from build123d import *

# Parameters (mm, degrees)
F2_DEPTH = 1
F1_R     = 0.25
F3_DEPTH = 25


with BuildPart() as f2:
    # F0 (on Top) → F2 (new body)
    with BuildSketch(Plane.XY):
        with BuildLine():
            ThreePointArc((30.5, 6.5), (28.010408, 12.510408), (22, 15))
            Line((22, 15), (-22, 15))
            ThreePointArc((-22, 15), (-28.010408, 12.510408), (-30.5, 6.5))
            Line((-30.5, 6.5), (-30.5, -6.5))
            ThreePointArc((-30.5, -6.5), (-28.010408, -12.510408), (-22, -15))
            Line((-22, -15), (22, -15))
            ThreePointArc((22, -15), (28.010408, -12.510408), (30.5, -6.5))
            Line((30.5, -6.5), (30.5, 6.5))
        make_face()
    extrude(amount=F2_DEPTH)

    # F1 (on face) → F3 (cut)
    with BuildSketch(Plane.XY):
        with Locations((-27.111111, 12)):
            Circle(F1_R)
        with Locations((-27.111111, 6)):
            Circle(F1_R)
        with Locations((-27.111111, 0)):
            Circle(F1_R)
        with Locations((-27.111111, -6)):
            Circle(F1_R)
        with Locations((-27.111111, -12)):
            Circle(F1_R)
        with Locations((-20.333333, 12)):
            Circle(F1_R)
        with Locations((-20.333333, 6)):
            Circle(F1_R)
        with Locations((-20.333333, 0)):
            Circle(F1_R)
        with Locations((-20.333333, -6)):
            Circle(F1_R)
        with Locations((-20.333333, -12)):
            Circle(F1_R)
        with Locations((-13.555556, 12)):
            Circle(F1_R)
        with Locations((-13.555556, 6)):
            Circle(F1_R)
        with Locations((-13.555556, 0)):
            Circle(F1_R)
        with Locations((-13.555556, -6)):
            Circle(F1_R)
        with Locations((-13.555556, -12)):
            Circle(F1_R)
        with Locations((-6.777778, 12)):
            Circle(F1_R)
        with Locations((-6.777778, 6)):
            Circle(F1_R)
        with Locations((-6.777778, 0)):
            Circle(F1_R)
        with Locations((-6.777778, -6)):
            Circle(F1_R)
        with Locations((-6.777778, -12)):
            Circle(F1_R)
        with Locations((0, 12)):
            Circle(F1_R)
        with Locations((0, 6)):
            Circle(F1_R)
        with Locations((0, 0)):
            Circle(F1_R)
        with Locations((0, -6)):
            Circle(F1_R)
        with Locations((0, -12)):
            Circle(F1_R)
        with Locations((6.777778, 12)):
            Circle(F1_R)
        with Locations((6.777778, 6)):
            Circle(F1_R)
        with Locations((6.777778, 0)):
            Circle(F1_R)
        with Locations((6.777778, -6)):
            Circle(F1_R)
        with Locations((6.777778, -12)):
            Circle(F1_R)
        with Locations((13.555556, 12)):
            Circle(F1_R)
        with Locations((13.555556, 6)):
            Circle(F1_R)
        with Locations((13.555556, 0)):
            Circle(F1_R)
        with Locations((13.555556, -6)):
            Circle(F1_R)
        with Locations((13.555556, -12)):
            Circle(F1_R)
        with Locations((20.333333, 12)):
            Circle(F1_R)
        with Locations((20.333333, 6)):
            Circle(F1_R)
        with Locations((20.333333, 0)):
            Circle(F1_R)
        with Locations((20.333333, -6)):
            Circle(F1_R)
        with Locations((20.333333, -12)):
            Circle(F1_R)
        with Locations((27.111111, 12)):
            Circle(F1_R)
        with Locations((27.111111, 6)):
            Circle(F1_R)
        with Locations((27.111111, 0)):
            Circle(F1_R)
        with Locations((27.111111, -6)):
            Circle(F1_R)
        with Locations((27.111111, -12)):
            Circle(F1_R)
    extrude(amount=F3_DEPTH, mode=Mode.SUBTRACT)


solid = f2.part
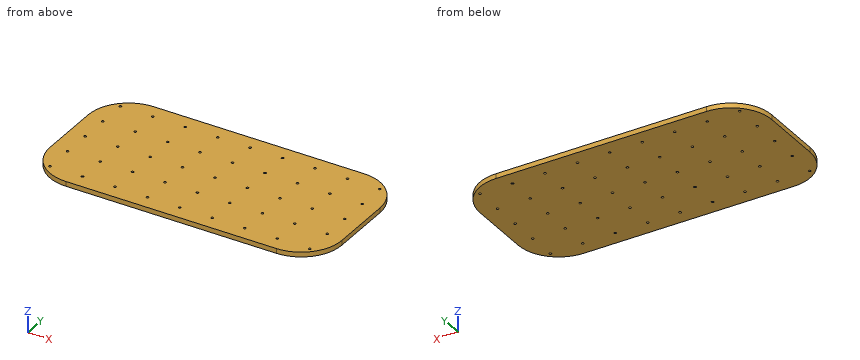
Geometry check sheet. Reference: the model listing, model coordinates, mm. Round coordinates to 2 decimals unless told otherwise and drop trailing zeros. Loops run counter-clockwise (first coordinate to the right, second up) from the corner with the lowest first, then second, coordinate; pieces in that order, holes last. Notation, with made-up numbers: (-30.75, 47.5) -> (5.25, 47.5) arc R26 ccw to (5.25, 77.5) -> close; hole circle Ø11 at (73, -26). An arc over 180 degrees is marked (long way). Answer as a JSON object with one key per item and string values. Group by question number.
Item 1: Cross-section at B-B, the plane y = -13. Record the cut outline in (x, z).
Item 2: Cross-section at A-A, the plane z = 0.7. Count the separate pieces of the cut face and the enclosed holes in it, plus the area to 3 significant figures.
Item 3: Thickness scan on line 1 along Y through (x, z) = (13.5, 0.55); line 2 along Y through (x, z) = (28, 0.8); line 3 along X through (y, z) = (-10, 0.2). Record the ranges inside material, lowest first.
Determined:
{
 "1": {"outline": "(-27.48, 0) -> (27.48, 0) -> (27.48, 1) -> (-27.48, 1) -> close"},
 "2": {"separate pieces": "1", "enclosed holes": "45", "area": "1,760 mm²"},
 "3": {"line 1": "y = -15 to -12.24, -11.76 to -6.24, -5.76 to -0.24, 0.24 to 5.76, 6.24 to 11.76, 12.24 to 15", "line 2": "y = -12.52 to 12.52", "line 3": "x = -29.75 to 29.75"}
}
